The figure shows three views and two pictorial views of one solid part (mm, origin at its lowest corner). Answer the questions. Coordinates: 2 decimals unless noted, no trailing zeros. Order: outer loops, then holes, each group sorted by start corner. A loop starts at its lowest first (then second) coordinate and runs counter-clockwise, first axis right, second up. Notation, with made-up numbers: (80.25, 14) -> (138.25, 14) arc R15 cw to (138.25, 18) -> close; hole circle Ø10 at (62, -11). An arc over 180 degrees is marked (long way). Return JSON: item names as keys, results as strings.
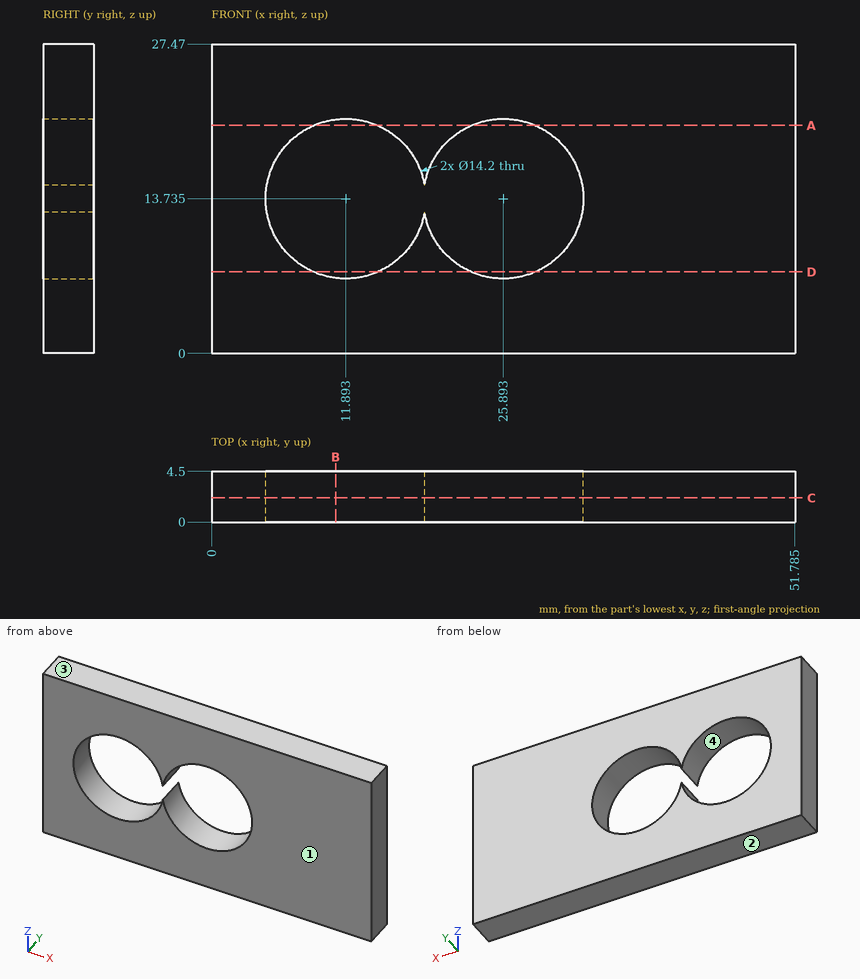
1. The part is cut by section D-D on z = 7.25. Give the vertices of the cut face in (x, y) (1 decimal), and give its area (3 significant figures).
Answer block:
{"outline": "(0, 0) -> (9, 0) -> (9, 4.5) -> (0, 4.5) -> close; (14.8, 0) -> (23, 0) -> (23, 4.5) -> (14.8, 4.5) -> close; (28.8, 0) -> (51.8, 0) -> (51.8, 4.5) -> (28.8, 4.5) -> close", "area": "181 mm2"}
2. The part is cut by section C-C on y = 2.15. Give the vertices of the cut face in (x, z) (1 decimal).
Answer block:
{"outline": "(0, 0) -> (51.8, 0) -> (51.8, 27.5) -> (0, 27.5) -> close; hole (18.9, 12.5) arc R7.1 ccw (long way) to (18.9, 14.9) arc R7.1 ccw (long way) to start"}
3. Consider line 1 (X direction, y = 4.05, z = 18.5) (1 decimal); line 2 (X direction, y = 3.7, z = 17) (1 decimal); line 3 (Z direction, x = 11.5, y = 1.1) (1 decimal). Determine where each line is inside the solid, lowest interval first. Write a range as from..to.
Answer block:
{"line 1": "x = 0..6.6, 17.2..20.6, 31.2..51.8", "line 2": "x = 0..5.6, 18.2..19.6, 32.2..51.8", "line 3": "z = 0..6.6, 20.8..27.5"}
4. The part is cut by section A-A on z = 20.25. Give the vertices of the cut face in (x, y) (1 decimal).
Answer block:
{"outline": "(0, 0) -> (9.1, 0) -> (9.1, 4.5) -> (0, 4.5) -> close; (14.7, 0) -> (23.1, 0) -> (23.1, 4.5) -> (14.7, 4.5) -> close; (28.7, 0) -> (51.8, 0) -> (51.8, 4.5) -> (28.7, 4.5) -> close"}
5. The part is cut by section B-B on x = 11. Give the vertices of the cut face in (y, z).
Answer block:
{"outline": "(0, 0) -> (4.5, 0) -> (4.5, 6.69) -> (0, 6.69) -> close; (0, 20.78) -> (4.5, 20.78) -> (4.5, 27.47) -> (0, 27.47) -> close"}
6. Determine the mould class of the marked faces 1, 2, 3 and 4 for opening direction Z: pulls with the +Z half, pulls with the -Z half, needs draft (parallel to the pull), parting line crosses it, or undercut.
Answer block:
{"face 1": "needs draft", "face 2": "pulls with the -Z half", "face 3": "pulls with the +Z half", "face 4": "undercut"}
